Verification items for the finished model (mm, model axes). A direction names the side the tool comes from. Give positions to 0.01 mm unless a question says otherwise; leave off trailing zeros. Order: outer loops, then holes, each group sorted by start corner. A loop starts at its lowest first (then second) coordinate and runs counter-clockwise, first axis right, second up. Notation, with made-up numbers: (-30, -20) - (11, -20) arc R9 cw to (11, -11) - close; hole circle Ø8 at (65.25, -6.75). An arc over 180 degrees is marked (long way). Answer as a JSON object with one key per item and string values.
```python
from build123d import *

# Parameters (mm, degrees)
SKETCH1_W           = 30
SKETCH1_H           = 123
SKETCH1_R           = 2.5
BOSS_EXTRUDE1_DEPTH = 3.175
FILLET2_R           = 5


with BuildPart() as part:
    # Sketch1 → Boss-Extrude1 (new body)
    with BuildSketch(Plane.XY):
        with Locations((0, 61.5)):
            Rectangle(SKETCH1_W, SKETCH1_H)
        with Locations((-8, 8)):
            Circle(SKETCH1_R, mode=Mode.SUBTRACT)
        with Locations(Location((8, 8, 0), (0, 0, 180))):
            Circle(SKETCH1_R, mode=Mode.SUBTRACT)
        with BuildLine():
            Line((2.5, 113), (2.5, 73))
            ThreePointArc((2.5, 73), (0, 70.5), (-2.5, 73))
            Line((-2.5, 73), (-2.5, 113))
            ThreePointArc((-2.5, 113), (0, 115.5), (2.5, 113))
        make_face(mode=Mode.SUBTRACT)
        with BuildLine():
            Line((-2.5, 63), (-2.5, 23))
            ThreePointArc((-2.5, 23), (0, 20.5), (2.5, 23))
            Line((2.5, 23), (2.5, 63))
            ThreePointArc((2.5, 63), (0, 65.5), (-2.5, 63))
        make_face(mode=Mode.SUBTRACT)
    extrude(amount=BOSS_EXTRUDE1_DEPTH)

    # Fillet2
    fillet2_edges = [part.edges().sort_by_distance(p)[0] for p in [
        (15, 123, 1.5875),
        (15, 0, 1.5875),
        (-15, 0, 1.5875),
        (-15, 123, 1.5875),
    ]]
    fillet(fillet2_edges, radius=FILLET2_R)


solid = part.part
```
(1) Section check A-A (y = 8). Record the cut outline in (x, z) (3 decimals), then the cut area to 3 significant figures.
Computed values:
{"outline": "(-15, 0) - (-10.5, 0) - (-10.5, 3.175) - (-15, 3.175) - close; (-5.5, 0) - (5.5, 0) - (5.5, 3.175) - (-5.5, 3.175) - close; (10.5, 0) - (15, 0) - (15, 3.175) - (10.5, 3.175) - close", "area": "63.5 mm²"}
(2) Section check C-C (z = 1.1). Record the cut outline in (x, y), then the cut area to 3 significant figures.
Computed values:
{"outline": "(-15, 5) arc R5 ccw to (-10, 0) - (10, 0) arc R5 ccw to (15, 5) - (15, 118) arc R5 ccw to (10, 123) - (-10, 123) arc R5 ccw to (-15, 118) - close; hole circle Ø5 at (-8, 8); hole (-2.5, 23) arc R2.5 ccw to (2.5, 23) - (2.5, 63) arc R2.5 ccw to (-2.5, 63) - close; hole (-2.5, 73) arc R2.5 ccw to (2.5, 73) - (2.5, 113) arc R2.5 ccw to (-2.5, 113) - close; hole circle Ø5 at (8, 8)", "area": "3,190 mm²"}
(3) Section check B-B (x = 0). Record the cut outline in (y, z) (3 decimals), then the cut area to 3 significant figures.
Computed values:
{"outline": "(0, 0) - (20.5, 0) - (20.5, 3.175) - (0, 3.175) - close; (65.5, 0) - (70.5, 0) - (70.5, 3.175) - (65.5, 3.175) - close; (115.5, 0) - (123, 0) - (123, 3.175) - (115.5, 3.175) - close", "area": "105 mm²"}
(4) Release check for a two-part mould opening along X. For faces 1 (the cylindrical face through (13, 1, 2)), 2 (the flat face through (0, 0, 2)), 3 (the cylindrical face through (-0.1, 20.5, 1.6)) record: pulls with the +X half, pulls with the -X half, needs draft (parallel to the pull), parting line crosses it, or undercut.
Computed values:
{"face 1": "pulls with the +X half", "face 2": "needs draft", "face 3": "undercut"}
(5) Section check D-D (y = 24.5). Record the cut outline in (x, z) (3 decimals).
Computed values:
{"outline": "(-15, 0) - (-2.5, 0) - (-2.5, 3.175) - (-15, 3.175) - close; (2.5, 0) - (15, 0) - (15, 3.175) - (2.5, 3.175) - close"}
(6) Access from +Z, -Z, +X, -X, +Y, -Y to the whole of each face (thin tool, end or side, straight path). Record for faces 4 (the flat face through (-2.5, 93, 2)), 5 (the flat face through (-4, 62, 0)).
Computed values:
{"face 4": "+Z, -Z", "face 5": "-Z, +X, -X, +Y, -Y"}
(7) Material ranges on line 1 along X through (y, z) = (50, 0.65); line 2 along Y through (x, z) = (-1, 2.45); line 3 along Y through (x, z) = (-8, 0.85), recorded low to high. Write a range as [from, to].
Computed values:
{"line 1": "x = [-15, -2.5], [2.5, 15]", "line 2": "y = [0, 20.71], [65.29, 70.71], [115.29, 123]", "line 3": "y = [0, 5.5], [10.5, 123]"}
